Build history of the part. All positions in model axes, mm. A direction names the side the tool comes from. Round coordinates to 2 decimals unless told otherwise and drop trailing zeros. Order: outer loops, then holes, each group sorted by start corner. A loop starts at its lowest first (then second) coordinate and runs counter-clockwise, first axis right, second up. Notation, with made-up numbers: (54, 39.25) -> (108, 39.25) arc R15 ccw to (108, 67.25) -> close; hole circle Ø4 at (86.5, 89.5). An arc over 180 degrees is marked (long way). Answer as a JSON object with one key per item and string values.
from build123d import *

# Parameters (mm, degrees)
SKETCH1_R           = 4
BOSS_EXTRUDE1_DEPTH = 4
SKETCH2_R           = 2.44
BOSS_EXTRUDE2_DEPTH = 6.55
SKETCH3_R           = 2.75
CUT_EXTRUDE1_DEPTH  = 3
SKETCH4_R           = 1.6
CUT_EXTRUDE2_DEPTH  = 10.434113631


with BuildPart() as part:
    # Sketch1 → Boss-Extrude1 (new body)
    with BuildSketch(Plane(origin=(0, 0, 0), x_dir=(1, 0, 0), z_dir=(0, 1, 0))):
        with Locations(Location((0, 0, 0), (0, 0, 270))):
            Circle(SKETCH1_R)
    extrude(amount=BOSS_EXTRUDE1_DEPTH)

    # Sketch2 → Boss-Extrude2 (add)
    with BuildSketch(Plane.XZ):
        with Locations(Location((0, 0, 0), (0, 0, 270))):
            Circle(SKETCH2_R)
    extrude(amount=BOSS_EXTRUDE2_DEPTH)

    # Sketch3 → Cut-Extrude1 (cut)
    with BuildSketch(Plane(origin=(0, 4, 0), x_dir=(1, 0, 0), z_dir=(0, 1, 0))):
        with Locations(Location((0, 0, 0), (0, 0, 270))):
            Circle(SKETCH3_R)
    extrude(amount=-CUT_EXTRUDE1_DEPTH, mode=Mode.SUBTRACT)

    # Sketch4 → Cut-Extrude2 (cut, through all)
    with BuildSketch(Plane(origin=(0, 1, 0), x_dir=(1, 0, 0), z_dir=(0, 1, 0))):
        with Locations(Location((0, 0, 0), (0, 0, 270))):
            Circle(SKETCH4_R)
    extrude(amount=-CUT_EXTRUDE2_DEPTH, mode=Mode.SUBTRACT)


solid = part.part
1) Cut at A-A, the plane x = 0. Give the cut face in (y, z), plus the area to 3 significant figures.
Checked values:
{"outline": "(-6.55, -2.44) -> (0, -2.44) -> (0, -4) -> (4, -4) -> (4, -2.75) -> (1, -2.75) -> (1, -1.6) -> (-6.55, -1.6) -> close; (-6.55, 1.6) -> (1, 1.6) -> (1, 2.75) -> (4, 2.75) -> (4, 4) -> (0, 4) -> (0, 2.44) -> (-6.55, 2.44) -> close", "area": "23.3 mm²"}
2) Cut at B-B, the plane z = 0. Give the cut face in (x, y), plus the area to 3 significant figures.
Checked values:
{"outline": "(-4, 0) -> (-2.44, 0) -> (-2.44, -6.55) -> (-1.6, -6.55) -> (-1.6, 1) -> (-2.75, 1) -> (-2.75, 4) -> (-4, 4) -> close; (1.6, -6.55) -> (2.44, -6.55) -> (2.44, 0) -> (4, 0) -> (4, 4) -> (2.75, 4) -> (2.75, 1) -> (1.6, 1) -> close", "area": "23.3 mm²"}
3) Which spindle directions (+Z, -Z, +X, -X, +Y, -Y) get a long thin tool onto all of the face, cutting with end or side? Do faces 1 (the face through (2, 0, 2)), 2 (the face through (-3.905, 1.972, -0.867)), 3 (the face through (-2.685, 2.521, -0.596)). Say none if no direction does.
Checked values:
{"face 1": "-Y", "face 2": "+Y, -Y", "face 3": "+Y"}
4) Cut at D-D, the plane y = -0.5. Give the cut face in (x, z).
Checked values:
{"outline": "circle Ø4.88 at (0, 0); hole circle Ø3.2 at (0, 0)"}
5) Cut at C-C, the plane y = 2. Give the cut face in (x, z), plus the area to 3 significant figures.
Checked values:
{"outline": "circle Ø8 at (0, 0); hole circle Ø5.5 at (0, 0)", "area": "26.5 mm²"}
6) Pull direction Z, two halves, no side cores. Call faces 4 (the face through (0, 1, 2)), 5 (the face through (-1.48, -3.23, 1.94)), 6 (the face through (-1, -6.55, -2)): pulls with the +Z half, pulls with the -Z half, needs draft (parallel to the pull), parting line crosses it, or undercut.
Checked values:
{"face 4": "undercut", "face 5": "parting line crosses it", "face 6": "needs draft"}
7) Probe L1, parallel to X at y = -3, z = 0; L2, parallel to Y at x = 2.5, z = 2; L3, parallel to Y at x = 0.75, z = 2.25. List the from-to ranges inside material, lowest first. Write a range as from..to.
Checked values:
{"L1": "x = -2.44..-1.6, 1.6..2.44", "L2": "y = 0..4", "L3": "y = -6.55..1"}
8) Flat gauge pins, fed straight in: pin 1 Ø4.5 at (x, z) = (0, 0) entering from +Y; pin 2 Ø1.5 at (y, z) = (-4, 0) entering from -X. Where does each tip first touch, or does it go through?
Checked values:
{"pin 1": "stops at y = 1", "pin 2": "stops at x = -2.44"}
